Check sheet for the drawn part. Datum: minimum x, y, z corner. Units: mm. Coordinates: 2 decimals unless noted, no trailing zeros. Loops run counter-clockwise (first coordinate to the right, second up) from the corner with the lowest first, then second, coordinate; pieces in that order, holes last.
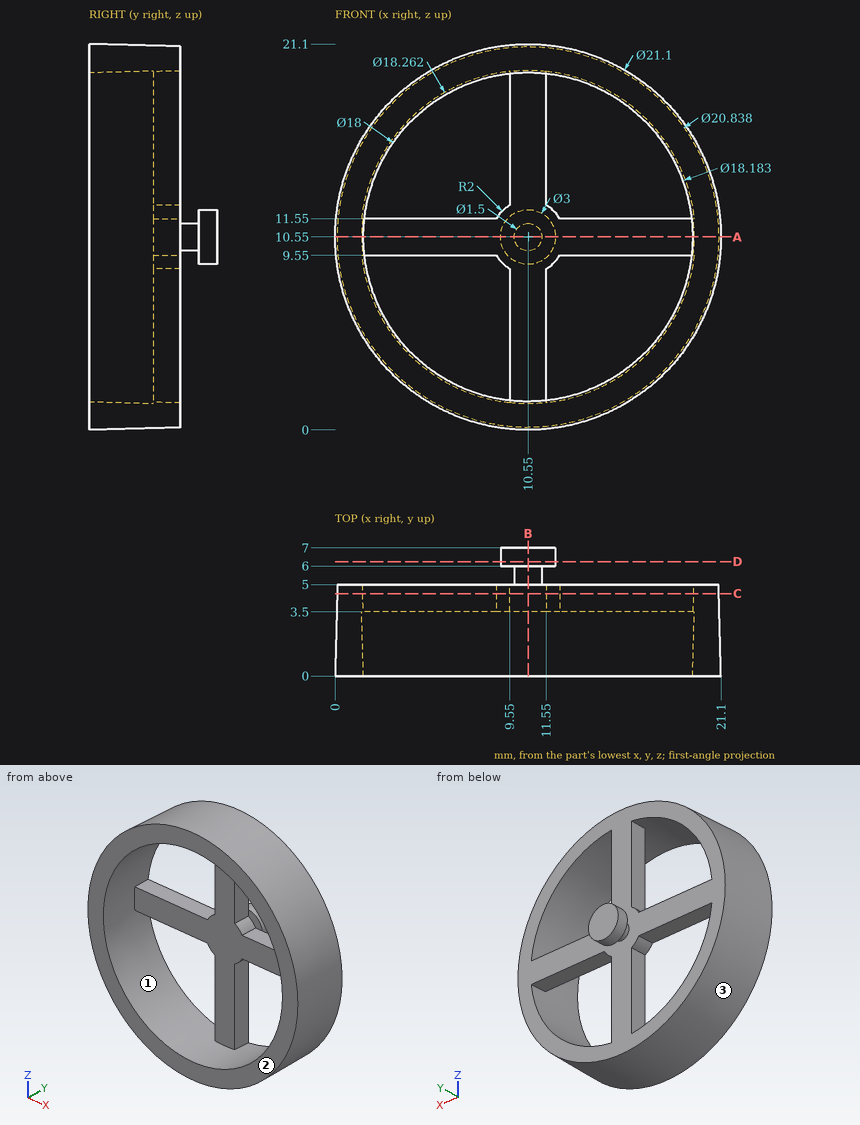
1) Scan lines: line 1 (Y direction, x = 3, z = 4); line 2 (Z direction, x = 8, y = 4.25); line 3 (Z direction, x = 3.5, y = 2.25). Record each from-to range of solid material in increasing order.
Answer sheet:
line 1: y = 0 to 5
line 2: z = 0.43 to 1.8, 9.55 to 11.55, 19.3 to 20.67
line 3: z = 2.78 to 4.86, 16.24 to 18.32
2) Mould release check, pull along Z, two halves, no side actions. Record for the marked faces 1, 2 and 3: +Z half, -Z half, draft (parallel to the pull), parting line (faces both ways), or undercut.
Answer sheet:
face 1: undercut
face 2: draft
face 3: parting line
3) Section check B-B on x = 10.55. Enter the section's corners in (y, z).
Answer sheet:
outline: (0, 0) - (5, 0.13) - (5, 9.8) - (6, 9.8) - (6, 9.05) - (7, 9.05) - (7, 12.05) - (6, 12.05) - (6, 11.3) - (5, 11.3) - (5, 20.97) - (0, 21.1) - (0, 19.55) - (3.5, 19.64) - (3.5, 1.46) - (0, 1.55) - close
4) Section check D-D on y = 6.25. Enter the section's corners in (x, z).
Answer sheet:
outline: circle Ø3 at (10.55, 10.55)
5) Section check A-A on z = 10.55. Enter the section's corners in (x, y).
Answer sheet:
outline: (0, 0) - (1.55, 0) - (1.46, 3.5) - (19.64, 3.5) - (19.55, 0) - (21.1, 0) - (20.97, 5) - (11.3, 5) - (11.3, 6) - (12.05, 6) - (12.05, 7) - (9.05, 7) - (9.05, 6) - (9.8, 6) - (9.8, 5) - (0.13, 5) - close
6) Section check C-C on y = 4.5. Enter the section's corners in (x, z), plus the area to 3 significant figures.
Answer sheet:
outline: circle Ø20.86 at (10.55, 10.55); hole (1.49, 9.55) arc R9.12 ccw to (9.55, 1.49) - (9.55, 8.82) arc R2 cw to (8.82, 9.55) - close; hole (1.49, 11.55) - (8.82, 11.55) arc R2 cw to (9.55, 12.28) - (9.55, 19.61) arc R9.12 ccw to start; hole (11.55, 1.49) arc R9.12 ccw to (19.61, 9.55) - (12.28, 9.55) arc R2 cw to (11.55, 8.82) - close; hole (11.55, 12.28) arc R2 cw to (12.28, 11.55) - (19.61, 11.55) arc R9.12 ccw to (11.55, 19.61) - close
area: 151 mm2
7) Depth check by flat-ended pin: pin 1 (3 mm diameter, centred on x = 15.5, z = 11, fed in from -Y); pin 2 (3 mm diameter, centred on x = 12, y = 5, fed in from -Z); pin 3 (1.2 mm diameter, centred on x = 15.5, y = 4.5, fed in from -Z). Enter the tip coordinate at first touch or a pass-through.
Answer sheet:
pin 1: stops at y = 3.5
pin 2: stops at z = 0.11
pin 3: stops at z = 1.07
